from build123d import *

# Parameters (mm, degrees)
SKETCH4_R           = 9.3853
SKETCH4_R_2         = 4.5847
BOSS_EXTRUDE1_DEPTH = 4.7498
SKETCH5_R           = 15.07617
BOSS_EXTRUDE2_DEPTH = 75.48314015
SKETCH6_R           = 4.5847
CUT_EXTRUDE1_DEPTH  = 158.168951984


with BuildPart() as part:
    # Sketch4 → Boss-Extrude1 (new body)
    with BuildSketch(Plane(origin=(0, 0, 0), x_dir=(0, 0, -1), z_dir=(1, 0, 0))):
        Circle(SKETCH4_R)
        Circle(SKETCH4_R_2, mode=Mode.SUBTRACT)
    boss_extrude1 = extrude(amount=BOSS_EXTRUDE1_DEPTH)

    # Sketch5 → Boss-Extrude2 (add)
    with BuildSketch(Plane(origin=(4.7498, 0, 0), x_dir=(0, 0, -1), z_dir=(1, 0, 0))):
        Circle(SKETCH5_R)
    boss_extrude2 = extrude(amount=BOSS_EXTRUDE2_DEPTH)

    # Mirror3: Boss-Extrude2 across plane
    add(boss_extrude2.mirror(Plane(origin=(80.23294015, 0, 0), x_dir=(0, 0, 1), z_dir=(1, 0, 0))))

    # Mirror4: Boss-Extrude1 across plane
    add(boss_extrude1.mirror(Plane(origin=(80.23294015, 0, 0), x_dir=(0, 0, 1), z_dir=(1, 0, 0))))

    # Sketch6 → Cut-Extrude1 (cut, through all)
    with BuildSketch(Plane(origin=(155.7160803, 0, 0), x_dir=(0, 0, -1), z_dir=(1, 0, 0))):
        Circle(SKETCH6_R)
    extrude(amount=-CUT_EXTRUDE1_DEPTH, mode=Mode.SUBTRACT)


solid = part.part
CAD build for the part. Positions are in the model's coordinates, mm. A direction names the side the tool comes from. Give positions to 0.01 mm unless a question says otherwise; leave off trailing zeros. Write each loop counter-clockwise with the first axis right and the second up, starting at its lowest first coordinate (ties: lowest second). Pieces come first, ordered by that corner, then holes. Notation, with made-up numbers: (10.5, -39.75) -> (32.5, -39.75) arc R29 ccw to (32.5, -9.75) -> close; hole circle Ø8 at (-14, 79). An arc over 180 degrees is marked (long way). Return JSON: item names as keys, results as strings.
Item 1: Drill centre lines: probe 1 along Y at (x, z) = (1.6, 0); probe 2 along Y at (x, z) = (39, 0); probe 3 along X at (y, z) = (-1.5, 12.5). Where is each one in solid material? Low to high.
Answer below:
{"probe 1": "y = -9.39 to -4.58, 4.58 to 9.39", "probe 2": "y = -15.08 to -4.58, 4.58 to 15.08", "probe 3": "x = 4.75 to 155.72"}
Item 2: Band-saw the part on D-D (y = -13). List the corners of the cut face in (x, z).
Answer below:
{"outline": "(4.75, -7.63) -> (155.72, -7.63) -> (155.72, 7.63) -> (4.75, 7.63) -> close"}
Item 3: Drop flat-ended pins along their axis: pin 1 (12 mm diameter, centred on x = 135.5, y = -7.5, fed in from -Z); pin 2 (8 mm diameter, centred on x = 90, y = -4.5, fed in from -Z); pin 3 (6 mm diameter, centred on x = 111.5, z = 9, fed in from -Y). Give the stop position or say it passes through.
Answer below:
{"pin 1": "stops at z = -15", "pin 2": "stops at z = -15.07", "pin 3": "stops at y = -13.83"}
Item 4: Band-saw the part on C-C (x = 109). List the corners of the cut face in (y, z).
Answer below:
{"outline": "circle Ø30.15 at (0, 0); hole circle Ø9.17 at (0, 0)"}
Item 5: Tool access for faces 1 (the cylindrical face through (158.124, 9.305, 1.222)), 2 (the cylindrical face through (2.342, 9.305, 1.222)), 3 (the flat face through (0, -2, 4.3)): list every direction of +Z, -Z, +X, -X, +Y, -Y with a clear straight run to the whole face (end or side of a thin tool).
Answer below:
{"face 1": "+X", "face 2": "-X", "face 3": "+Z, -Z, -X, +Y, -Y"}
Item 6: Band-saw the part on A-A (y = 0). List the corners of the cut face in (x, z), then the cut area to 3 significant figures.
Answer below:
{"outline": "(0, -9.39) -> (4.75, -9.39) -> (4.75, -15.08) -> (155.72, -15.08) -> (155.72, -9.39) -> (160.47, -9.39) -> (160.47, -4.58) -> (0, -4.58) -> close; (0, 4.58) -> (160.47, 4.58) -> (160.47, 9.39) -> (155.72, 9.39) -> (155.72, 15.08) -> (4.75, 15.08) -> (4.75, 9.39) -> (0, 9.39) -> close", "area": "3,260 mm2"}
